Geometry check sheet. Reference: the model listing, model coordinates, mm. Coordinates: 2 decimals unless noted, no trailing zeros. Loops run counter-clockwise (first coordinate to the right, second up) from the corner with the lowest first, then second, coordinate; pieces in that order, holes last.
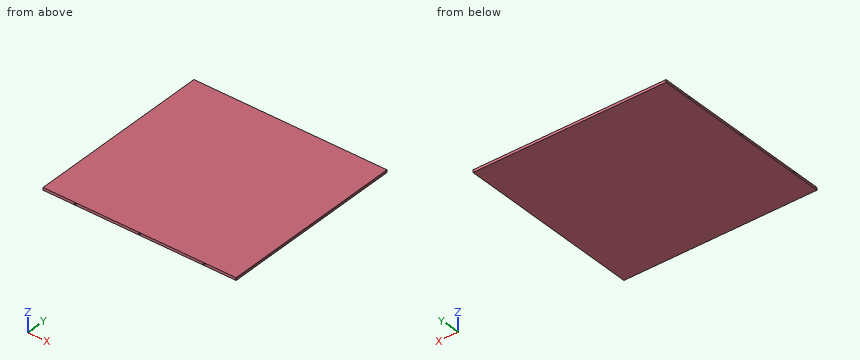
from build123d import *

# Parameters (mm, degrees)
SKETCH1_W           = 300
SKETCH1_H           = 300
BOSS_EXTRUDE1_DEPTH = 4
SKETCH2_R           = 1.5
CUT_EXTRUDE1_DEPTH  = 25
SKETCH3_W           = 300
SKETCH3_H           = 10
CUT_EXTRUDE2_DEPTH  = 5
SKETCH4_R           = 1.5
CUT_EXTRUDE3_DEPTH  = 25


with BuildPart() as part:
    # Sketch1 → Boss-Extrude1 (new body)
    with BuildSketch(Plane.XY):
        with Locations((150, 150)):
            Rectangle(SKETCH1_W, SKETCH1_H)
    extrude(amount=BOSS_EXTRUDE1_DEPTH)

    # Sketch2 → Cut-Extrude1 (cut)
    with BuildSketch(Plane(origin=(0, 0, 0), x_dir=(-1, 0, 0), z_dir=(0, -1, 0))):
        with Locations((-50, -2)):
            Circle(SKETCH2_R)
        with Locations((-250, -2)):
            Circle(SKETCH2_R)
        with Locations((-150, -2)):
            Circle(SKETCH2_R)
    extrude(amount=-CUT_EXTRUDE1_DEPTH, mode=Mode.SUBTRACT)

    # Sketch3 → Cut-Extrude2 (cut, through all)
    with BuildSketch(Plane(origin=(0, 0, 0), x_dir=(-1, 0, 0), z_dir=(0, 0, -1))):
        with Locations((-150, 295)):
            Rectangle(SKETCH3_W, SKETCH3_H)
    extrude(amount=-CUT_EXTRUDE2_DEPTH, mode=Mode.SUBTRACT)

    # Sketch4 → Cut-Extrude3 (cut)
    with BuildSketch(Plane.ZY):
        with Locations((2, 245)):
            Circle(SKETCH4_R)
        with Locations((2, 45)):
            Circle(SKETCH4_R)
        with Locations((2, 145)):
            Circle(SKETCH4_R)
    extrude(amount=-CUT_EXTRUDE3_DEPTH, mode=Mode.SUBTRACT)


solid = part.part
(1) Gauge pin test, flat ends, axial feed: pin 1 Ø1.5 at (y, z) = (144.5, 2) entering from -X; pin 2 Ø1.5 at (x, y) = (167.5, 179.5) entering from -Z. Record the tip position at first contact, or that the pin passes through.
Findings:
pin 1: stops at x = 25
pin 2: stops at z = 0
(2) Sectioned sample at A-A on x = 20. Record the cut outline in (y, z), and give its area (3 significant figures).
Findings:
outline: (0, 0) - (290, 0) - (290, 4) - (0, 4) - close; hole circle Ø3 at (45, 2); hole circle Ø3 at (145, 2); hole circle Ø3 at (245, 2)
area: 1,140 mm2
(3) Scan lines: L1, parallel to X at y = 9.5, z = 2; L2, parallel to Z at x = 50, y = 7; L3, parallel to Y at x = 50, z = 2.85. Record each from-to range of solid material in increasing order.
Findings:
L1: x = 0 to 48.5, 51.5 to 148.5, 151.5 to 248.5, 251.5 to 300
L2: z = 0 to 0.5, 3.5 to 4
L3: y = 25 to 290
